Source: CAD feature listing. Evaluate the final solid. Frame: model axes, mm. A direction names the side the tool comes from. Give positions to 0.01 mm unless a question says otherwise; leave off trailing zeros. Order: outer loops, then holes, each group sorted by start corner. A loop starts at its lowest first (then second) coordinate and runs counter-clockwise, first axis right, second up. Notation, with made-up numbers: M 74.25,76.25 L 85.25,76.25 A24 ccw 85.25,107.25 Z; hole C -34,44.25 d1. An arc over 180 degrees is marked long. Answer in a Markdown table with one row per item. Add a question column.
(1) Pin query (flat end, axial travel): P1, Ø7.5, axis at y = 15.5, z = 13.5, coming from the +X side; P2, Ø10, axis at x = -26, y = 8.5, coming from the +Z side; P3, Ø12, axis at y = 11, z = 32.5, coming from the -X side; P4, Ø8, axis at x = -39.5, z = 37, coming from the +Y side. Return the tip coordinate at first contact, or that it passes through.
(2) Section query A-A, the plane z = 11.5. Return loops of the section in (x, y).
(3) Section query C-C, the plane x = 13. Return loops of the section in (y, z).
(4) Material intervals for line 1 along X through (y, z) = (8.5, 22); line 2 along Z through (x, y) = (9, -8.5), sorted ascending.
(5) Set-up query: faces 1 (the face through (-50.8, -13, 26)), 2 (the face through (-13, 25.4, 13)), 3 (the face through (13, 0, 13)), 4 (the face through (-25.4, 13, 13)), 5 (the face through (-25.4, -13, 38)). Return all of +Z, -Z, +X, -X, +Y, -Y with unobstructed straight access to the full face (end or side cutting, diameter ignored); none if empty.
(6) Section query B-B, the plane y = -5.5. Return loops of the section in (x, z).
from build123d import *

# Parameters (mm, degrees)
F0_W     = 25.4
F0_H     = 25.4
F1_DEPTH = 25.4
F2_W     = 25.4
F2_H     = 25.4
F3_DEPTH = 25.4


with BuildPart() as f1:
    # F0 (on Front) → F1 (new body)
    with BuildSketch(Plane.XZ):
        with Locations((-38.1, 12.7)):
            Rectangle(F0_W, F0_H)
        with Locations((-12.7, 12.7)):
            Rectangle(F0_W, F0_H)
        with Locations((12.7, 12.7)):
            Rectangle(F0_W, F0_H)
        with Locations((-38.1, 38.1)):
            Rectangle(F0_W, F0_H)
    extrude(amount=F1_DEPTH)

    # F2 (on Top) → F3 (join)
    with BuildSketch(Plane.XY):
        with Locations((-12.7, 12.7)):
            Rectangle(F2_W, F2_H)
    extrude(amount=F3_DEPTH)


solid = f1.part
Values follow:
| question | item | result |
|---|---|---|
| 1 | P1 | stops at x = 0 |
| 1 | P2 | stops at z = 25.4 |
| 1 | P3 | passes through |
| 1 | P4 | stops at y = 0 |
| 2 | outline | M -50.8,-25.4 L 25.4,-25.4 L 25.4,0 L 0,0 L 0,25.4 L -25.4,25.4 L -25.4,0 L -50.8,0 Z |
| 3 | outline | M -25.4,0 L 0,0 L 0,25.4 L -25.4,25.4 Z |
| 4 | line 1 | x = -25.4 to 0 |
| 4 | line 2 | z = 0 to 25.4 |
| 5 | face 1 | +Z, -Z, -X, +Y, -Y |
| 5 | face 2 | +Z, -Z, +X, -X, +Y |
| 5 | face 3 | +Z, -Z, +X, +Y |
| 5 | face 4 | +Z, -Z, -X, +Y |
| 5 | face 5 | +Z, +X, +Y, -Y |
| 6 | outline | M -50.8,0 L 25.4,0 L 25.4,25.4 L -25.4,25.4 L -25.4,50.8 L -50.8,50.8 Z |
